```python
from build123d import *


with BuildPart() as part:
    # Esquisse1 → Révolution1 (revolve)
    with BuildSketch(Plane.XY, mode=Mode.PRIVATE) as r_volution1_sk:
        Polygon((-5, 2.75), (-2, 2.75), (-2, 6.25), (0, 6.25), (0, 9.5), (-3.5, 9.5), (-5.5, 6.75), (-12, 6.75), (-12, 5.25), (-5, 5.25), align=None)
    revolve(r_volution1_sk.sketch.rotate(Axis((-19.911160568, 0, 0), (1, 0, 0)), 90), axis=Axis((-19.911160568, 0, 0), (1, 0, 0)))  # turned: the seam where the file's is


solid = part.part
```
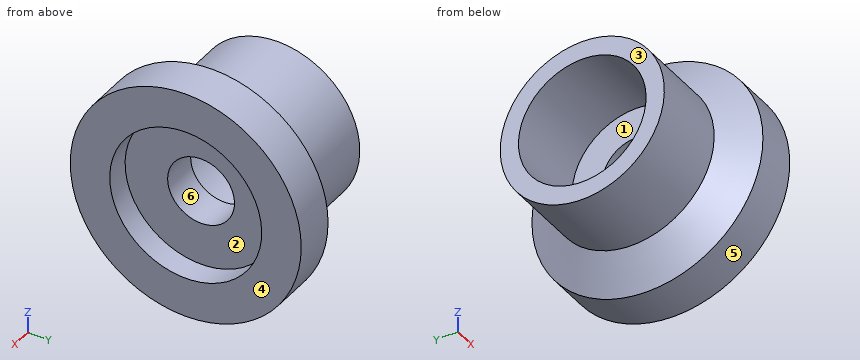
Design review of the part built by this model. Coordinates are the model's own, in mm. Face numbers are marked on the shaded views. A direction names the side the tool comes from. Give positions to 0.01 mm unless a question says otherwise; leave off trailing zeros. Order: outer loops, then holes, each group sorted by start corner. A loop starts at its lowest first (then second) coordinate and runs counter-clockwise, first axis right, second up. Notation, with made-up numbers: (62.5, -39.75) -> (79.5, -39.75) arc R12 cw to (79.5, -20.75) -> close; hole circle Ø3 at (-30, 61.5). An arc over 180 degrees is marked (long way). Write each question's results on one line, items separated by ' | '. Start each with the question number.
Q1. Wall thickness on L1, parallel to Y at x = -0.9, z = 0; L2, parallel to Y at x = -10, z = 0; L3, parallel to X at y = 4.25, z = 0.5: over which ranges is each line inside the solid? List them lowest first. Write a range as from..to.
Q2. Machinability: for the marked faces 1, 2 and 3, which of the approach directions +Z, -Z, +X, -X, +Y, -Y give a long, thin tool a straight path to every point of the face, cutting with its end or side? Answer none if there is none.
Q3. For pin 1 (9 mm diameter, centred on y = 0, z = 0, fed in from -X); pin 2 (5 mm diameter, centred on x = -10, y = -5, fed in from -Z); pin 3 (4 mm diameter, centred on x = -6.5, z = 2.5, fed in from +Y), all flat-tipped, find the tip position at first contact; note any pin that passes through.
Q4. Add section C-C on x = -1.25. Give the boundary of the cut face in (y, z).
Q5. Mouldability with a two-part tool opening along Z and no side actions: class the marked faces 4, 5 and 6 as +Z half, -Z half, draft (parallel to the pull), parting line (faces both ways), or undercut.
Q6. Add section D-D on x = -3.25. Give the boundary of the cut face in (y, z).
Q7. Add section A-A on y = 0. Give the boundary of the cut face in (x, z), and give its area (4 significant figures).
Found:
1) L1: y = -9.5..-6.25, 6.25..9.5 | L2: y = -6.75..-5.25, 5.25..6.75 | L3: x = -5..-2
2) face 1: -X | face 2: +X | face 3: +Z, -Z, -X, +Y, -Y
3) pin 1: stops at x = -5 | pin 2: stops at z = -6.27 | pin 3: stops at y = 7.79
4) outline: circle Ø19 at (0, 0); hole circle Ø12.5 at (0, 0)
5) face 4: draft | face 5: parting line | face 6: undercut
6) outline: circle Ø19 at (0, 0); hole circle Ø5.5 at (0, 0)
7) outline: (-12, -6.75) -> (-5.5, -6.75) -> (-3.5, -9.5) -> (0, -9.5) -> (0, -6.25) -> (-2, -6.25) -> (-2, -2.75) -> (-5, -2.75) -> (-5, -5.25) -> (-12, -5.25) -> close; (-12, 5.25) -> (-5, 5.25) -> (-5, 2.75) -> (-2, 2.75) -> (-2, 6.25) -> (0, 6.25) -> (0, 9.5) -> (-3.5, 9.5) -> (-5.5, 6.75) -> (-12, 6.75) -> close | area: 71.75 mm2
